Build history of the part. All positions in model axes, mm. Give positions to 0.01 mm unless a question says otherwise; leave off trailing zeros. Order: outer loops, then holes, each group sorted by start corner. A loop starts at its lowest first (then second) coordinate and runs counter-clockwise, first axis right, second up. Notation, with made-up numbers: M 8,70.25 L 37,70.25 A24 cw 37,97.25 Z; hole C 62,18 d3. An arc over 180 degrees is marked long. Answer as CSV lines item,"result".
from build123d import *

# Parameters (mm, degrees)
SKIZZE1_W                       = 410
SKIZZE1_H                       = 410
AUFSATZ_LINEAR_AUSTRAGEN1_DEPTH = 5
SKIZZE2_W                       = 97.796702903
SKIZZE2_H                       = 49.6
SCHNITT_LINEAR_AUSTRAGEN1_DEPTH = 5
LINEARES_MUSTER1_COUNT          = 4
LINEARES_MUSTER1_PITCH          = 99.9
SPIEGELN1_COPY_1_SKETCH_W       = 97.796702903
SPIEGELN1_COPY_1_SKETCH_H       = 49.6
SPIEGELN1_COPY_1_DEPTH          = 5
SPIEGELN1_COPY_2_SKETCH_W       = 97.796702903
SPIEGELN1_COPY_2_SKETCH_H       = 49.6
SPIEGELN1_COPY_2_DEPTH          = 5
SPIEGELN1_COPY_3_SKETCH_W       = 97.796702903
SPIEGELN1_COPY_3_SKETCH_H       = 49.6
SPIEGELN1_COPY_3_DEPTH          = 5
SKIZZE3_W                       = 49.6
SKIZZE3_H                       = 41.77912255
SCHNITT_LINEAR_AUSTRAGEN2_DEPTH = 5
LINEARES_MUSTER2_COUNT          = 4
LINEARES_MUSTER2_PITCH          = 99.9
SPIEGELN2_COPY_1_SKETCH_W       = 49.6
SPIEGELN2_COPY_1_SKETCH_H       = 41.77912255
SPIEGELN2_COPY_1_DEPTH          = 5
SPIEGELN2_COPY_2_SKETCH_W       = 49.6
SPIEGELN2_COPY_2_SKETCH_H       = 41.77912255
SPIEGELN2_COPY_2_DEPTH          = 5
SPIEGELN2_COPY_3_SKETCH_W       = 49.6
SPIEGELN2_COPY_3_SKETCH_H       = 41.77912255
SPIEGELN2_COPY_3_DEPTH          = 5
SCHNITT_LINEAR_AUSTRAGEN3_DEPTH = 5
SPIEGELN4_COPY_1_DEPTH          = 5
SCHNITT_LINEAR_AUSTRAGEN4_REACH = 581.849
SKIZZE5_R                       = 57.5
SKIZZE5_R_2                     = 2
SKIZZE5_3_R                     = 2
SCHNITT_LINEAR_AUSTRAGEN5_DEPTH = 10


with BuildPart() as part:
    # Skizze1 → Aufsatz-Linear austragen1 (new body)
    with BuildSketch(Plane.XY):
        with Locations((205, 205)):
            Rectangle(SKIZZE1_W, SKIZZE1_H)
    extrude(amount=AUFSATZ_LINEAR_AUSTRAGEN1_DEPTH)

    # Skizze2 → Schnitt-Linear austragen1 (cut)
    with BuildSketch(Plane.XY.offset(5)):
        with Locations((-43.898351452, 354.85)):
            Rectangle(SKIZZE2_W, SKIZZE2_H)
    schnitt_linear_austragen1 = extrude(amount=-SCHNITT_LINEAR_AUSTRAGEN1_DEPTH, mode=Mode.SUBTRACT)

    # Lineares Muster1: Schnitt-Linear austragen1 ×4
    with Locations(*[(0, -i * LINEARES_MUSTER1_PITCH, 0) for i in range(1, LINEARES_MUSTER1_COUNT)]):
        add(schnitt_linear_austragen1, mode=Mode.SUBTRACT)

    # Spiegeln1: Schnitt-Linear austragen1 across plane
    add(schnitt_linear_austragen1.mirror(Plane(origin=(205, 0, 0), x_dir=(0, 0, 1), z_dir=(1, 0, 0))), mode=Mode.SUBTRACT)

    # Spiegeln1 copy 1 sketch → Spiegeln1 copy 1 (cut)
    with BuildSketch(Plane(origin=(410, -99.9, 5), x_dir=(-1, 0, 0), z_dir=(0, 0, 1))):
        with Locations((-43.898351452, -354.85)):
            Rectangle(SPIEGELN1_COPY_1_SKETCH_W, SPIEGELN1_COPY_1_SKETCH_H)
    extrude(amount=-SPIEGELN1_COPY_1_DEPTH, mode=Mode.SUBTRACT)

    # Spiegeln1 copy 2 sketch → Spiegeln1 copy 2 (cut)
    with BuildSketch(Plane(origin=(410, -199.8, 5), x_dir=(-1, 0, 0), z_dir=(0, 0, 1))):
        with Locations((-43.898351452, -354.85)):
            Rectangle(SPIEGELN1_COPY_2_SKETCH_W, SPIEGELN1_COPY_2_SKETCH_H)
    extrude(amount=-SPIEGELN1_COPY_2_DEPTH, mode=Mode.SUBTRACT)

    # Spiegeln1 copy 3 sketch → Spiegeln1 copy 3 (cut)
    with BuildSketch(Plane(origin=(410, -299.7, 5), x_dir=(-1, 0, 0), z_dir=(0, 0, 1))):
        with Locations((-43.898351452, -354.85)):
            Rectangle(SPIEGELN1_COPY_3_SKETCH_W, SPIEGELN1_COPY_3_SKETCH_H)
    extrude(amount=-SPIEGELN1_COPY_3_DEPTH, mode=Mode.SUBTRACT)

    # Skizze3 → Schnitt-Linear austragen2 (cut)
    with BuildSketch(Plane.XY.offset(5)):
        with Locations((55.15, 425.889561275)):
            Rectangle(SKIZZE3_W, SKIZZE3_H)
    schnitt_linear_austragen2 = extrude(amount=-SCHNITT_LINEAR_AUSTRAGEN2_DEPTH, mode=Mode.SUBTRACT)

    # Lineares Muster2: Schnitt-Linear austragen2 ×4
    with Locations(*[(i * LINEARES_MUSTER2_PITCH, 0, 0) for i in range(1, LINEARES_MUSTER2_COUNT)]):
        add(schnitt_linear_austragen2, mode=Mode.SUBTRACT)

    # Spiegeln2: Schnitt-Linear austragen2 across plane
    add(schnitt_linear_austragen2.mirror(Plane.ZX.offset(205)), mode=Mode.SUBTRACT)

    # Spiegeln2 copy 1 sketch → Spiegeln2 copy 1 (cut)
    with BuildSketch(Plane(origin=(99.9, 410, 5), x_dir=(1, 0, 0), z_dir=(0, 0, 1))):
        with Locations((55.15, -425.889561275)):
            Rectangle(SPIEGELN2_COPY_1_SKETCH_W, SPIEGELN2_COPY_1_SKETCH_H)
    extrude(amount=-SPIEGELN2_COPY_1_DEPTH, mode=Mode.SUBTRACT)

    # Spiegeln2 copy 2 sketch → Spiegeln2 copy 2 (cut)
    with BuildSketch(Plane(origin=(199.8, 410, 5), x_dir=(1, 0, 0), z_dir=(0, 0, 1))):
        with Locations((55.15, -425.889561275)):
            Rectangle(SPIEGELN2_COPY_2_SKETCH_W, SPIEGELN2_COPY_2_SKETCH_H)
    extrude(amount=-SPIEGELN2_COPY_2_DEPTH, mode=Mode.SUBTRACT)

    # Spiegeln2 copy 3 sketch → Spiegeln2 copy 3 (cut)
    with BuildSketch(Plane(origin=(299.7, 410, 5), x_dir=(1, 0, 0), z_dir=(0, 0, 1))):
        with Locations((55.15, -425.889561275)):
            Rectangle(SPIEGELN2_COPY_3_SKETCH_W, SPIEGELN2_COPY_3_SKETCH_H)
    extrude(amount=-SPIEGELN2_COPY_3_DEPTH, mode=Mode.SUBTRACT)

    # Skizze4 → Schnitt-Linear austragen3 (cut)
    with BuildSketch(Plane.XY.offset(5)):
        Polygon((5, 379.65), (5, 405), (30.35, 405), (30.35, 431.549801047), (5, 431.549801047), (-47.862925009, 431.549801047), (-47.862925009, 405), (-47.862925009, 379.65), align=None)
    schnitt_linear_austragen3 = extrude(amount=-SCHNITT_LINEAR_AUSTRAGEN3_DEPTH, mode=Mode.SUBTRACT)

    # Spiegeln3: Schnitt-Linear austragen3 across plane
    add(schnitt_linear_austragen3.mirror(Plane(origin=(205, 0, 0), x_dir=(0, 0, 1), z_dir=(1, 0, 0))), mode=Mode.SUBTRACT)

    # Spiegeln4: Schnitt-Linear austragen3 across plane
    add(schnitt_linear_austragen3.mirror(Plane.ZX.offset(205)), mode=Mode.SUBTRACT)

    # Spiegeln4 copy 1 sketch → Spiegeln4 copy 1 (cut)
    with BuildSketch(Plane(origin=(410, 410, 5), x_dir=(-1, 0, 0), z_dir=(0, 0, 1))):
        Polygon((5, 379.65), (5, 405), (30.35, 405), (30.35, 431.549801047), (5, 431.549801047), (-47.862925009, 431.549801047), (-47.862925009, 405), (-47.862925009, 379.65), align=None)
    extrude(amount=-SPIEGELN4_COPY_1_DEPTH, mode=Mode.SUBTRACT)

    # Skizze5 → Schnitt-Linear austragen4 (cut, up to next)
    with BuildSketch(Plane(origin=(0, 0, 0), x_dir=(-1, 0, 0), z_dir=(0, 0, -1)), mode=Mode.PRIVATE) as schnitt_linear_austragen4_sk1:
        with Locations((-340, 255)):
            Circle(SKIZZE5_R)
    schnitt_linear_austragen4_tool1 = extrude(schnitt_linear_austragen4_sk1.sketch, amount=-SCHNITT_LINEAR_AUSTRAGEN4_REACH, mode=Mode.PRIVATE) & part.part
    # Skizze5 → Schnitt-Linear austragen4 (cut, up to next)
    with BuildSketch(Plane(origin=(0, 0, 0), x_dir=(-1, 0, 0), z_dir=(0, 0, -1)), mode=Mode.PRIVATE) as schnitt_linear_austragen4_sk2:
        with Locations((-287.5, 307.5)):
            Circle(SKIZZE5_R_2)
    schnitt_linear_austragen4_tool2 = extrude(schnitt_linear_austragen4_sk2.sketch, amount=-SCHNITT_LINEAR_AUSTRAGEN4_REACH, mode=Mode.PRIVATE) & part.part
    # Skizze5 → Schnitt-Linear austragen4 (cut, up to next)
    with BuildSketch(Plane(origin=(0, 0, 0), x_dir=(-1, 0, 0), z_dir=(0, 0, -1)), mode=Mode.PRIVATE) as schnitt_linear_austragen4_sk3:
        with Locations((-392.5, 202.5)):
            Circle(SKIZZE5_R_2)
    schnitt_linear_austragen4_tool3 = extrude(schnitt_linear_austragen4_sk3.sketch, amount=-SCHNITT_LINEAR_AUSTRAGEN4_REACH, mode=Mode.PRIVATE) & part.part
    # Skizze5 → Schnitt-Linear austragen4 (cut, up to next)
    with BuildSketch(Plane(origin=(0, 0, 0), x_dir=(-1, 0, 0), z_dir=(0, 0, -1)), mode=Mode.PRIVATE) as schnitt_linear_austragen4_sk4:
        with Locations((-392.5, 307.5)):
            Circle(SKIZZE5_R_2)
    schnitt_linear_austragen4_tool4 = extrude(schnitt_linear_austragen4_sk4.sketch, amount=-SCHNITT_LINEAR_AUSTRAGEN4_REACH, mode=Mode.PRIVATE) & part.part
    # Skizze5 → Schnitt-Linear austragen4 (cut, up to next)
    with BuildSketch(Plane(origin=(0, 0, 0), x_dir=(-1, 0, 0), z_dir=(0, 0, -1)), mode=Mode.PRIVATE) as schnitt_linear_austragen4_sk5:
        with Locations((-287.5, 202.5)):
            Circle(SKIZZE5_R_2)
    schnitt_linear_austragen4_tool5 = extrude(schnitt_linear_austragen4_sk5.sketch, amount=-SCHNITT_LINEAR_AUSTRAGEN4_REACH, mode=Mode.PRIVATE) & part.part
    schnitt_linear_austragen4_1 = schnitt_linear_austragen4_tool1.solids().sort_by_distance((340, 255, 0))[0]
    add(schnitt_linear_austragen4_1, mode=Mode.SUBTRACT)
    schnitt_linear_austragen4_2 = schnitt_linear_austragen4_tool2.solids().sort_by_distance((287.5, 307.5, 0))[0]
    add(schnitt_linear_austragen4_2, mode=Mode.SUBTRACT)
    schnitt_linear_austragen4_3 = schnitt_linear_austragen4_tool3.solids().sort_by_distance((392.5, 202.5, 0))[0]
    add(schnitt_linear_austragen4_3, mode=Mode.SUBTRACT)
    schnitt_linear_austragen4_4 = schnitt_linear_austragen4_tool4.solids().sort_by_distance((392.5, 307.5, 0))[0]
    add(schnitt_linear_austragen4_4, mode=Mode.SUBTRACT)
    schnitt_linear_austragen4_5 = schnitt_linear_austragen4_tool5.solids().sort_by_distance((287.5, 202.5, 0))[0]
    add(schnitt_linear_austragen4_5, mode=Mode.SUBTRACT)
    schnitt_linear_austragen4 = schnitt_linear_austragen4_1 + schnitt_linear_austragen4_2 + schnitt_linear_austragen4_3 + schnitt_linear_austragen4_4 + schnitt_linear_austragen4_5  # Schnitt-Linear austragen4 as one shape, for the pattern or mirror that repeats it

    # Skizze5<3> → Schnitt-Linear austragen5 (cut)
    with BuildSketch(Plane(origin=(0, 0, 0), x_dir=(-1, 0, 0), z_dir=(0, 0, -1))):
        with Locations((-350, 139.5)):
            Circle(SKIZZE5_3_R)
        with Locations((-160, 139.5)):
            Circle(SKIZZE5_3_R)
        with Locations((-160, 30.5)):
            Circle(SKIZZE5_3_R)
        with Locations((-350, 30.5)):
            Circle(SKIZZE5_3_R)
        with BuildLine():
            Line((-339, 125), (-171, 125))
            ThreePointArc((-171, 125), (-170.292893219, 124.707106781), (-170, 124))
            Line((-170, 124), (-170, 46))
            ThreePointArc((-170, 46), (-170.292893219, 45.292893219), (-171, 45))
            Line((-171, 45), (-339, 45))
            ThreePointArc((-339, 45), (-339.707106781, 45.292893219), (-340, 46))
            Line((-340, 46), (-340, 124))
            ThreePointArc((-340, 124), (-339.707106781, 124.707106781), (-339, 125))
        make_face()
    extrude(amount=-SCHNITT_LINEAR_AUSTRAGEN5_DEPTH, mode=Mode.SUBTRACT)

    # Spiegeln5: Schnitt-Linear austragen4 across plane
    add(schnitt_linear_austragen4.mirror(Plane(origin=(205, 0, 0), x_dir=(0, 0, 1), z_dir=(1, 0, 0))), mode=Mode.SUBTRACT)


solid = part.part
Item 1: Band-saw the part on B-B (x = 70). Give the cut face in (y, z), and give its area (4 significant figures).
Geometry says:
outline,"M 5,0 L 197.5,0 L 197.5,5 L 5,5 Z; M 312.5,0 L 405,0 L 405,5 L 312.5,5 Z"
area,"1,425 mm2"
Item 2: Band-saw the part on D-D (x = 295.5). Give the cut face in (y, z).
Geometry says:
outline,"M 0,0 L 45,0 L 45,5 L 0,5 Z; M 125,0 L 218.59,0 L 218.59,5 L 125,5 Z; M 291.41,0 L 410,0 L 410,5 L 291.41,5 Z"
Item 3: Probe line 1 along Y through (x, z) = (160, 2.95); line 2 along Y through (x, z) = (338.5, 2.7); line 3 along Y through (x, z) = (287.5, 2.55). List the from-to ranges inside material, lowest first. Write a range as from..to.
Geometry says:
line 1,"y = 5..28.5, 32.5..137.5, 141.5..405"
line 2,"y = 5..45, 125..197.52, 312.48..405"
line 3,"y = 0..45, 125..200.5, 204.5..231.55, 278.45..305.5, 309.5..410"
Item 4: Drop flat-ended pins along their axis: pin 1 (2.5 mm diameter, centred on y = 3, z = 1.5, fed in from +X); pin 2 (1.5 mm diameter, centred on x = 352.5, z = 2, fed in from +Y); pin 3 (1.5 mm diameter, centred on y = 172, z = 2, fed in from -X). Give the stop position or say it passes through.
Geometry says:
pin 1,"stops at x = 330.05"
pin 2,"stops at y = 405"
pin 3,"stops at x = 5"
Item 5: Band-saw the part on C-C (y = 255). Give the cut face in (x, z), and give its area (3 significant figures).
Geometry says:
outline,"M 5,0 L 12.5,0 L 12.5,5 L 5,5 Z; M 127.5,0 L 282.5,0 L 282.5,5 L 127.5,5 Z; M 397.5,0 L 405,0 L 405,5 L 397.5,5 Z"
area,"850 mm2"
Item 6: Pull direction X, two halves, no side cores. Call faces 1 (the cylindrical face through (62.51, 312.01, 2.46)), 2 (the flat face through (202, 208, 0)), 3 (the cylindrical face through (285.155, 272.271, 2.465)): released by +X, released by -X, zero draft, split by the parting line, or undercut.
Geometry says:
face 1,"undercut"
face 2,"zero draft"
face 3,"undercut"
Item 7: Band-saw the part on A-A (y = 119). Give the cut face in (x, z).
Geometry says:
outline,"M 0,0 L 170,0 L 170,5 L 0,5 Z; M 340,0 L 410,0 L 410,5 L 340,5 Z"
